Verification items for the finished model (mm, model axes). A direction names the side the tool comes from. Coordinates: 2 decimals unless noted, no trailing zeros. Loops run counter-clockwise (first coordinate to the right, second up) from the corner with the lowest first, then second, coordinate; pieces in that order, holes last. Notation, with made-up numbers: (73.5, 76) -> (118.5, 76) arc R21 cw to (118.5, 108) -> close; hole circle Ø2 at (47.25, -21.75). An arc over 180 degrees is marked (long way). Write item = value, one per line.
Autodesk Inventor part; units mm, degrees
ref_plane "YZ Plane" through (0, 0, 0) normal (1, 0, 0) x (0, 1, 0)
ref_plane "XZ Plane" through (0, 0, 0) normal (0, 1, 0) x (-1, 0, 0)
ref_plane "XY Plane" through (0, 0, 0) normal (0, 0, 1) x (1, 0, 0)
sketch "Sketch1" plane through (0, 0, 0) normal (0, 1, 0) x (-1, 0, 0)
  line L0 (10.85, 0) -> (0, 0)
  line L1 (0, -9) -> (26, -9)
  line L2 (26, -9) -> (26, -1)
  circle A0 centre (15, 0) radius 4.15
  line L3 (19.0277, -1) -> (26, -1)
  line L4 (0, 9) -> (26, 9)
  line L5 (26, 9) -> (26, 1)
  circle A1 centre (15, 0) radius 4.15
  line L6 (19.0277, 1) -> (26, 1)
  line L7 (0, -9) -> (0, 0)
  line L8 (0, 9) -> (0, 0)
  point P0 (19.0277, 1)
  dimension "d2" = 1
  dimension "d3" = 9
  dimension "d4" = 8.3
  dimension "d27" = 15
  dimension "d28" = 26
extrude "Extrusion1" add sketch "Sketch1" along normal blind 10 contours A0 L3 L2 L1 L7 L0 | L0 L8 L4 L5 L6 A0
sketch "Sketch7" plane through (0, 10, 0) normal (0, 1, 0) x (1, 0, 0)
  line L0 (0, -9) -> (0, 9)
  line L1 (-31.2, 0) -> (5.2, 0)
  arc A0 (-19.0277, -1) -> (-19.0277, 1) centre (-15, 0) ccw
  point P0 (0, 0)
  point P1 (-6, -4)
  point P2 (0, 0)
  point P3 (-6, 4)
  dimension "d44" = 8
  dimension "d45" = 9
hole "Hole1" at (-6, 10, 4) at (-6, 10, -4) direction (0, -1, 0) diameter 3.3 end through all counterbore diameter 5.8 counterbore depth 2.7
sketch "Sketch3" plane through (0, 0, -9) normal (0, 0, -1) x (-1, 0, 0)
  circle A0 centre (21.9389, 5) radius 1.75
  line L0 (26, 0) -> (26, 10)
  line L1 (10.85, 10) -> (19.0277, 10)
  point P0 (0, 0)
  point P1 (26, 5)
  point P2 (14.9389, 10)
  dimension "d15" = 3.5
  dimension "d46" = 7
extrude "Extrusion3" cut sketch "Sketch3" against normal up to surface (18 mm away)
sketch "Sketch4" plane through (-26, 0, 9) normal (0, 0, 1) x (1, 0, 0)
  line L0 (1.1611, 6.6743) -> (4.0611, 8.3486)
  line L1 (4.0611, 8.3486) -> (6.9611, 6.6743)
  line L2 (6.9611, 6.6743) -> (6.9611, 3.3257)
  line L3 (6.9611, 3.3257) -> (4.0611, 1.6514)
  line L4 (4.0611, 1.6514) -> (1.1611, 3.3257)
  line L5 (1.1611, 3.3257) -> (1.1611, 6.6743)
  circle A0 centre (4.0611, 5) radius 1.75
  point P0 (26, 0)
  point P1 (1.1611, 5)
  dimension "d20" = 5.8
extrude "Extrusion4" cut sketch "Sketch4" against normal blind 3
sketch "Sketch5" plane through (0, 0, -9) normal (0, 0, -1) x (-1, 0, 0)
  circle A0 centre (21.9389, 5) radius 2.9
  circle A1 centre (21.9389, 5) radius 1.75
  point P0 (0, 0)
  dimension "d23" = 5.8
extrude "Extrusion5" cut sketch "Sketch5" against normal blind 2
chamfer "Chamfer1" distance 3 angle 45 2 edges at (0, 5, 9) (0, 5, -9)
equation "\"d17\" = d15"
properties part number "Shaft support"
1) Tool access check on faces 1 (the face through (-24.705, 5.871, -8.014)), 2 (the face through (-4, 7.3, -4)), 3 (the face through (-19.039, 5, 8)), 4 (the face through (-10.853, 4.93, -0.168)). Record the directions out of +Z, -Z, +X, -X, +Y, -Y that give a thin tool (end or side, any length) a straight path to the whole face; none if there is none.
Ans:
face_1 = -Z
face_2 = +Y
face_3 = +Z
face_4 = +Y, -Y
2) Release check for a two-part mould opening along Z. For faces 5 (the face through (-20.47, 2.5, 7.52)), 6 (the face through (-24, 5, -1)), 7 (the face through (-14, 5, -9)), 8 (the face through (-1, 5, 7)) record: pulls with the +Z half, pulls with the -Z half, needs draft (parallel to the pull), parting line crosses it, or undercut.
Ans:
face_5 = needs draft
face_6 = undercut
face_7 = pulls with the -Z half
face_8 = pulls with the +Z half
3) Depth check by flat-ended pin: pin 1 Ø2 at (x, y) = (-21.94, 5) entering from -Z; pin 2 Ø4.5 at (x, z) = (-6, 4) entering from +Y; pin 3 Ø4.5 at (x, y) = (-21.94, 5) entering from -Z. Enter the tip coordinate at first touch or a pass-through.
Ans:
pin_1 = through
pin_2 = 7.3
pin_3 = -7
4) Sectioned sample at A-A, the plane y = 5. Record the cut outline in (x, z), plus the area to 3 significant figures.
Ans:
outline = (-26, -9) -> (-24.84, -9) -> (-24.84, -7) -> (-23.69, -7) -> (-23.69, -1) -> (-26, -1) -> close; (-26, 1) -> (-23.69, 1) -> (-23.69, 6) -> (-24.84, 6) -> (-24.84, 9) -> (-26, 9) -> close; (-20.19, -7) -> (-19.04, -7) -> (-19.04, -9) -> (-3, -9) -> (0, -6) -> (0, 6) -> (-3, 9) -> (-19.04, 9) -> (-19.04, 6) -> (-20.19, 6) -> (-20.19, 1) -> (-19.03, 1) arc R4.15 cw (long way) to (-19.03, -1) -> (-20.19, -1) -> close; hole circle Ø3.3 at (-6, -4); hole circle Ø3.3 at (-6, 4)
area = 307 mm2
5) Material ranges on line 1 (Z direction, x = -6, y = 8.4); line 2 (Z direction, x = -4, y = 7.5); line 3 (Z direction, x = -22.5, y = 1), recorded low to high.
Ans:
line_1 = -9 to -6.9, -1.1 to 1.1, 6.9 to 9
line_2 = -9 to -6.1, -1.9 to 1.9, 6.1 to 9
line_3 = -9 to -1, 1 to 9
6) Sectioned sample at B-B, the plane z = -3. Record the cut outline in (x, y).
Ans:
outline = (-26, 0) -> (-17.87, 0) -> (-17.87, 10) -> (-26, 10) -> close; (-12.13, 0) -> (-7.31, 0) -> (-7.31, 7.3) -> (-8.72, 7.3) -> (-8.72, 10) -> (-12.13, 10) -> close; (-4.69, 0) -> (0, 0) -> (0, 10) -> (-3.28, 10) -> (-3.28, 7.3) -> (-4.69, 7.3) -> close; hole circle Ø3.5 at (-21.94, 5)
7) Sectioned sample at C-C, the plane x = -15. Record the cut outline in (y, z).
Ans:
outline = (0, -9) -> (10, -9) -> (10, -4.15) -> (0, -4.15) -> close; (0, 4.15) -> (10, 4.15) -> (10, 9) -> (0, 9) -> close
8) Sectioned sample at D-D, the plane y = 0.5. Record the cut outline in (x, z).
Ans:
outline = (-26, -9) -> (-3, -9) -> (0, -6) -> (0, 6) -> (-3, 9) -> (-26, 9) -> (-26, 1) -> (-19.03, 1) arc R4.15 cw (long way) to (-19.03, -1) -> (-26, -1) -> close; hole circle Ø3.3 at (-6, -4); hole circle Ø3.3 at (-6, 4)
